Read the model definition and answer for the solid it produces. Units are mm, in the model's axes. Face numbers are marked on the shaded views. Coordinates: 2 decimals unless noted, no trailing zeros. Write each loop counter-clockwise with the first axis right and the second up, starting at its lowest first coordinate (ties: lowest second). Pieces come first, ordered by that corner, then holes. Notation, with made-up numbers: (50.5, -28) - (99.5, -28) arc R25 cw to (99.5, 0) - close; hole circle Ø11 at (36, -38). An arc over 180 degrees is marked (long way). Use a Markdown table: item, result.
from build123d import *

# Parameters (mm, degrees)
SKETCH1_R                 = 45.95
BOSS_EXTRUDE1_DEPTH       = 3
SKETCH2_R                 = 45.95
SKETCH2_R_2               = 40.95
BOSS_EXTRUDE2_DEPTH       = 22.4
F_4_40_TAPPED_HOLE3_D     = 2.2606
F_4_40_TAPPED_HOLE3_DEPTH = 7.6
F_4_40_TAPPED_HOLE3_TIP   = 0.679152758
SKETCH11_R                = 1.5
CUT_EXTRUDE1_DEPTH        = 46.95
CUT_EXTRUDE1_DEPTH_BACK   = 46.95
SKETCH12_R                = 45.95
SKETCH12_R_2              = 40.95
BOSS_EXTRUDE3_DEPTH       = 25.4
SKETCH14_R                = 1.5
CUT_EXTRUDE2_DEPTH        = 46.95000011
CUT_EXTRUDE2_DEPTH_BACK   = 46.95000011
SKETCH15_R                = 3
CUT_EXTRUDE3_DEPTH        = 10


with BuildPart() as part:
    # Sketch1 → Boss-Extrude1 (new body)
    with BuildSketch(Plane(origin=(0, 0, 0), x_dir=(1, 0, 0), z_dir=(0, 1, 0))):
        Circle(SKETCH1_R)
    extrude(amount=BOSS_EXTRUDE1_DEPTH)

    # Sketch2 → Boss-Extrude2 (add)
    with BuildSketch(Plane(origin=(0, 3, 0), x_dir=(1, 0, 0), z_dir=(0, 1, 0))):
        Circle(SKETCH2_R)
        Circle(SKETCH2_R_2, mode=Mode.SUBTRACT)
    extrude(amount=BOSS_EXTRUDE2_DEPTH)

    # #4-40 Tapped Hole3
    with Locations(Plane(origin=(0, 0, 0), x_dir=(-1, 0, 0), z_dir=(0, -1, 0))):
        with Locations((9.5, 0), (4.75, -8.227241336), (-4.75, -8.227241336), (-9.5, 0), (-4.75, 8.227241336), (4.75, 8.227241336)):
            Hole(F_4_40_TAPPED_HOLE3_D / 2, depth=F_4_40_TAPPED_HOLE3_DEPTH)
            with Locations((0, 0, -(F_4_40_TAPPED_HOLE3_DEPTH + F_4_40_TAPPED_HOLE3_TIP / 2))):  # 118° drill point
                Cone(0, F_4_40_TAPPED_HOLE3_D / 2, F_4_40_TAPPED_HOLE3_TIP, mode=Mode.SUBTRACT)

    # Sketch11 → Cut-Extrude1 (cut, two sides)
    with BuildSketch(Plane.XY) as cut_extrude1_sk:
        with Locations((0, 13.9)):
            Circle(SKETCH11_R)
        with Locations((0, -13.9)):
            Circle(SKETCH11_R)
    extrude(amount=CUT_EXTRUDE1_DEPTH, mode=Mode.SUBTRACT)
    extrude(cut_extrude1_sk.sketch, amount=-CUT_EXTRUDE1_DEPTH_BACK, mode=Mode.SUBTRACT)

    # Sketch12 → Boss-Extrude3 (add)
    with BuildSketch(Plane(origin=(0, 25.4, 0), x_dir=(1, 0, 0), z_dir=(0, 1, 0))):
        Circle(SKETCH12_R)
        Circle(SKETCH12_R_2, mode=Mode.SUBTRACT)
    extrude(amount=BOSS_EXTRUDE3_DEPTH)

    # Sketch14 → Cut-Extrude2 (cut, two sides)
    with BuildSketch(Plane.XY) as cut_extrude2_sk:
        with Locations((0, 36.9)):
            Circle(SKETCH14_R)
    extrude(amount=CUT_EXTRUDE2_DEPTH, mode=Mode.SUBTRACT)
    extrude(cut_extrude2_sk.sketch, amount=-CUT_EXTRUDE2_DEPTH_BACK, mode=Mode.SUBTRACT)

    # Sketch15 → Cut-Extrude3 (cut)
    with BuildSketch(Plane(origin=(0, 3, 0), x_dir=(1, 0, 0), z_dir=(0, 1, 0))):
        Circle(SKETCH15_R)
    extrude(amount=-CUT_EXTRUDE3_DEPTH, mode=Mode.SUBTRACT)


solid = part.part
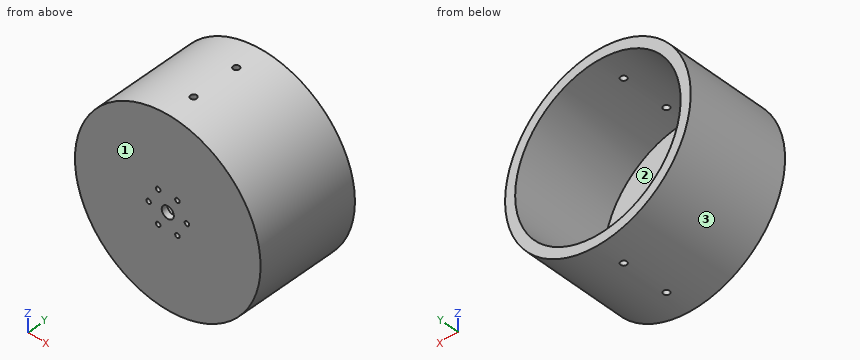
(1) A cutting plane is placed at B-B, the plane x = 0. Write down the section's boundary in (y, z), and give its area (3 significant figures).
Report:
| item | result |
|---|---|
| outline | (0, -45.95) - (12.4, -45.95) - (12.4, -40.95) - (3, -40.95) - (3, -3) - (0, -3) - close; (0, 3) - (3, 3) - (3, 40.95) - (12.4, 40.95) - (12.4, 45.95) - (0, 45.95) - close; (15.4, -45.95) - (35.4, -45.95) - (35.4, -40.95) - (15.4, -40.95) - close; (15.4, 40.95) - (35.4, 40.95) - (35.4, 45.95) - (15.4, 45.95) - close; (38.4, -45.95) - (50.8, -45.95) - (50.8, -40.95) - (38.4, -40.95) - close; (38.4, 40.95) - (50.8, 40.95) - (50.8, 45.95) - (38.4, 45.95) - close |
| area | 676 mm² |
(2) A cutting plane is placed at D-D, the plane z = 34. Write down the section's boundary in (x, y), and give its area (3 significant figures).
Report:
| item | result |
|---|---|
| outline | (-30.91, 0) - (30.91, 0) - (30.91, 50.8) - (22.82, 50.8) - (22.82, 3) - (-22.82, 3) - (-22.82, 50.8) - (-30.91, 50.8) - close |
| area | 959 mm² |
(3) The mould has two halves that part along X. Classify the marked faces 1, 2 and 3: pulls with the +X half, pulls with the -X half, needs draft (parallel to the pull), parting line crosses it, or undercut.
Report:
| item | result |
|---|---|
| face 1 | needs draft |
| face 2 | undercut |
| face 3 | parting line crosses it |
(4) A cutting plane is placed at A-A, the plane z = 0. Write down the section's boundary in (x, y), and give its area (3 significant figures).
Report:
| item | result |
|---|---|
| outline | (-45.95, 0) - (-10.63, 0) - (-10.63, 3) - (-40.95, 3) - (-40.95, 50.8) - (-45.95, 50.8) - close; (-8.37, 0) - (-3, 0) - (-3, 3) - (-8.37, 3) - close; (3, 0) - (8.37, 0) - (8.37, 3) - (3, 3) - close; (10.63, 0) - (45.95, 0) - (45.95, 50.8) - (40.95, 50.8) - (40.95, 3) - (10.63, 3) - close |
| area | 722 mm² |
(5) Each of these flat-tipped pins is pushed along its axis until it touches: P1, Ø8, axis at x = -35.5, y = 19.5, coming from the -Z side; P2, Ø2.5, axis at x = -4.75, z = 8.23, coming from the +Y side; P3, Ø10, axis at x = 22, y = 15.5, coming from the +Z side. Where does it stop, or does it pass through?
Report:
| item | result |
|---|---|
| P1 | stops at z = -33.45 |
| P2 | stops at y = 3 |
| P3 | stops at z = 42.69 |
(6) Straight lines are drawn through the part: L1, parallel to Y at x = 0, z = -44; L2, parallel to Z at x = 4.75, y = 1.25; L3, parallel to Y at x = -21.5, z = -30. For each, find the intervals that lie inside material, in ascending order.
Report:
| item | result |
|---|---|
| L1 | y = 0 to 12.4, 15.4 to 35.4, 38.4 to 50.8 |
| L2 | z = -45.7 to -9.36, -7.1 to 7.1, 9.36 to 45.7 |
| L3 | y = 0 to 3 |
